CAD build for the part. Positions are in the model's coordinates, mm. Face numbers are marked on the shaded views. A direction names the side the tool comes from. Coordinates: 2 decimals unless noted, no trailing zeros. Write each loop counter-clockwise with the first axis right and the second up, starting at its lowest first coordinate (ties: lowest second). Pieces come first, ordered by that corner, then holes. Notation, with made-up numbers: (16, -10) - (49, -10) arc R19 ccw to (49, 9) - close; hole circle Ø11 at (71.5, 43). An arc over 180 degrees is marked (long way). One line per question, with ' | ' between items. Start each with the question number.
1. Flat gauge pins, fed straight in: P1, Ø1.5, axis at y = -23, z = 7, coming from the +X side; P2, Ø5, axis at y = -28.5, z = 38.5, coming from the -X side; P3, Ø4, axis at y = -18, z = 40, coming from the +X side; P4, Ø10, axis at y = -26.5, z = 0.5, coming from the +X side. Where does each tip first touch, or does it go through?
2. Band-saw the part on A-A, the plane y = -19.05. Write the cut outline in (x, z).
3. Probe line 1 (Y direction, x = 15, z = 4); line 2 (Z direction, x = -14.5, y = -22.5); line 3 (X direction, y = -34, z = 28). List the from-to ranges inside material, lowest first.
4. Which spindle directions (+Z, -Z, +X, -X, +Y, -Y) get a long thin tool onto all of the face, cutting with end or side? Do the marked faces 4, 5 and 6. Say none if no direction does.
5. Band-saw the part on D-D, the plane y = -25. Write the cut outline in (x, z).
6. Band-saw the part on C-C, the plane y = -34. Write the cut outline in (x, z).
7. Band-saw the part on B-B, the plane x = 30.5. Write the cut outline in (y, z).
8. Two-plate mould, pull along Z, no slides. Class the marked faces 1, 2 and 3: +Z half, -Z half, draft (parallel to the pull), parting line (faces both ways), or undercut.
from build123d import *

# Parameters (mm, degrees)
F0_R     = 7.527389
F1_DEPTH = 38.1
F3_DEPTH = 14.789578
F4_DEPTH = 14.789578


with BuildPart() as f1:
    # F0 (on Front) → F1 (new body)
    with BuildSketch(Plane.XZ):
        with BuildLine():
            Line((-62.946253, -7.394289), (62.946253, -7.394289))
            Line((62.946253, -7.394289), (62.946253, 7.394289))
            Line((62.946253, 7.394289), (-35.454668, 7.394289))
            Line((-35.454668, 7.394289), (-35.454668, 38.109027))
            ThreePointArc((-35.454668, 38.109027), (-49.20046, 51.854819), (-62.946253, 38.109027))
            Line((-62.946253, 38.109027), (-62.946253, 7.394289))
            Line((-62.946253, 7.394289), (-62.946253, -7.394289))
        make_face()
        with Locations((-49.20046, 38.109027)):
            Circle(F0_R, mode=Mode.SUBTRACT)
    extrude(amount=F1_DEPTH)

    # F2 (on face) → F3 (cut, through all)
    with BuildSketch(Plane.XY.offset(7.394289)):
        with BuildLine():
            Line((0, -27.397288), (40.194597, -27.397288))
            ThreePointArc((40.194597, -27.397288), (48.541885, -19.05), (40.194597, -10.702712))
            Line((40.194597, -10.702712), (0, -10.702712))
            ThreePointArc((0, -10.702712), (-8.347288, -19.05), (0, -27.397288))
        make_face()
    extrude(amount=-F3_DEPTH, mode=Mode.SUBTRACT)

    # F2 (on face) → F4 (cut, through all)
    with BuildSketch(Plane.XY.offset(7.394289)):
        with BuildLine():
            Line((62.946253, 0), (40.194597, 0))
            ThreePointArc((40.194597, 0), (59.244597, -19.05), (40.194597, -38.1))
            Line((40.194597, -38.1), (62.946253, -38.1))
            Line((62.946253, -38.1), (62.946253, 0))
        make_face()
    extrude(amount=-F4_DEPTH, mode=Mode.SUBTRACT)


solid = f1.part
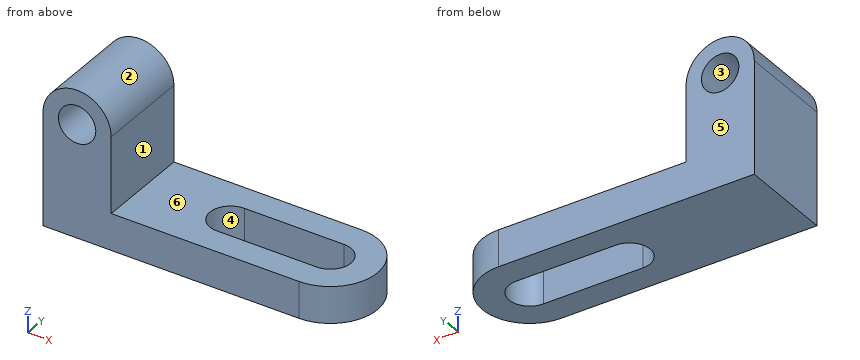
Filled in:
1) P1: stops at x = 58.97 | P2: stops at x = -62.95 | P3: stops at x = -35.45 | P4: stops at x = 59.09
2) outline: (-62.95, -7.39) - (-8.35, -7.39) - (-8.35, 7.39) - (-35.45, 7.39) - (-35.45, 38.11) arc R13.75 ccw to (-62.95, 38.11) - close; (48.54, -7.39) - (59.24, -7.39) - (59.24, 7.39) - (48.54, 7.39) - close; hole circle Ø15.05 at (-49.2, 38.11)
3) line 1: y = -38.1 to -27.4, -10.7 to 0 | line 2: z = -7.39 to 7.39 | line 3: x = -62.95 to -35.45
4) face 4: +Z, -Z | face 5: +Z, -Z, +X, -X, +Y | face 6: +Z, +X, +Y, -Y
5) outline: (-62.95, -7.39) - (-5.85, -7.39) - (-5.85, 7.39) - (-35.45, 7.39) - (-35.45, 38.11) arc R13.75 ccw to (-62.95, 38.11) - close; (46.05, -7.39) - (58.29, -7.39) - (58.29, 7.39) - (46.05, 7.39) - close; hole circle Ø15.05 at (-49.2, 38.11)
6) outline: (-62.95, -7.39) - (52, -7.39) - (52, 7.39) - (-35.45, 7.39) - (-35.45, 38.11) arc R13.75 ccw to (-62.95, 38.11) - close; hole circle Ø15.05 at (-49.2, 38.11)
7) outline: (-38.1, -7.39) - (-27.4, -7.39) - (-27.4, 7.39) - (-38.1, 7.39) - close; (-10.7, -7.39) - (0, -7.39) - (0, 7.39) - (-10.7, 7.39) - close
8) face 1: draft | face 2: +Z half | face 3: undercut
